The listing builds one solid part. Answer for the finished solid, in the listing's coordinates (mm). Face numbers are marked on the shaded views. A direction names the side the tool comes from. Coordinates: 2 decimals unless noted, no trailing zeros. Order: outer loops, then holes, each group sorted by start corner. A loop starts at its lowest first (then second) coordinate and runs counter-clockwise, first axis right, second up. Notation, with made-up numbers: (-13.75, 2.25) -> (13.25, 2.25) arc R22 cw to (13.25, 9.25) -> close; hole circle Ø4 at (76, 5). An arc over 180 degrees is marked (long way). One line per question, with ' | ' between items.
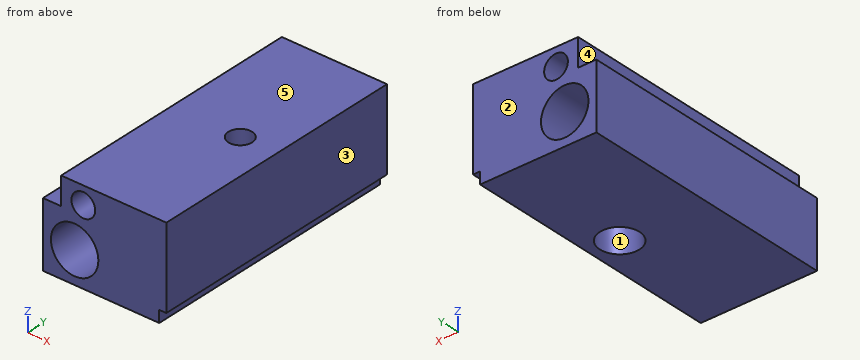
from build123d import *

# Parameters (mm, degrees)
F0_R          = 3
F0_R_2        = 1.5
F1_DEPTH      = 16.5
F1_DEPTH_BACK = 16.5
F2_R          = 1.5
F2_R_2        = 2.5
F3_DEPTH      = 6.5
F4_DEPTH      = 11.8


with BuildPart() as f1:
    # F0 (on Front) → F1 (new body, two sides)
    with BuildSketch(Plane.XZ) as f1_sk:
        Polygon((0, 8.3), (0, 0), (14.7, 0), (14.7, 1.5), (15.6, 1.5), (15.6, 11.8), (2.3, 11.8), (2.3, 8.3), align=None)
        with Locations((4, 4)):
            Circle(F0_R, mode=Mode.SUBTRACT)
        with Locations((5.1, 9.55)):
            Circle(F0_R_2, mode=Mode.SUBTRACT)
    extrude(amount=F1_DEPTH)
    extrude(f1_sk.sketch, amount=-F1_DEPTH_BACK)

    # F2 (on face) → F3 (cut)
    with BuildSketch(Plane(origin=(0, 0, 0), x_dir=(1, 0, 0), z_dir=(0, 0, -1))):
        with Locations((11, 0)):
            Circle(F2_R)
        with Locations((11, 0)):
            Circle(F2_R_2)
        with Locations((11, 0)):
            Circle(F2_R, mode=Mode.SUBTRACT)
    extrude(amount=-F3_DEPTH, mode=Mode.SUBTRACT)

    # F2 (on face) → F4 (cut, through all)
    with BuildSketch(Plane(origin=(0, 0, 0), x_dir=(1, 0, 0), z_dir=(0, 0, -1))):
        with Locations((11, 0)):
            Circle(F2_R)
    extrude(amount=-F4_DEPTH, mode=Mode.SUBTRACT)


solid = f1.part
Item 1: For the marked faces 4 and 5, determine the directions among +Z, -Z, +X, -X, +Y, -Y from which every point of the face is accessible in a straight line to the end or side of a thin tool.
Computed values:
face 4: +Z, -X, +Y, -Y | face 5: +Z, +X, -X, +Y, -Y
Item 2: Section C-C, the plane y = -1 is taken. Give the vertices of the cut face in (x, z), plus the area to 3 significant figures.
Computed values:
outline: (0, 0) -> (8.71, 0) -> (8.71, 6.5) -> (9.88, 6.5) -> (9.88, 11.8) -> (2.3, 11.8) -> (2.3, 8.3) -> (0, 8.3) -> close; (12.12, 6.5) -> (13.29, 6.5) -> (13.29, 0) -> (14.7, 0) -> (14.7, 1.5) -> (15.6, 1.5) -> (15.6, 11.8) -> (12.12, 11.8) -> close; hole circle Ø6 at (4, 4); hole circle Ø3 at (5.1, 9.55) | area: 97.7 mm^2
Item 3: Section B-B, the plane x = 11 is taken. Give the vertices of the cut face in (y, z), plus the area to 3 significant figures.
Computed values:
outline: (-16.5, 0) -> (-2.5, 0) -> (-2.5, 6.5) -> (-1.5, 6.5) -> (-1.5, 11.8) -> (-16.5, 11.8) -> close; (1.5, 6.5) -> (2.5, 6.5) -> (2.5, 0) -> (16.5, 0) -> (16.5, 11.8) -> (1.5, 11.8) -> close | area: 341 mm^2
Item 4: Section D-D, the plane x = 5 is taken. Give the vertices of the cut face in (y, z), plus the area to 3 significant figures.
Computed values:
outline: (-16.5, 0) -> (16.5, 0) -> (16.5, 1.17) -> (-16.5, 1.17) -> close; (-16.5, 6.83) -> (16.5, 6.83) -> (16.5, 8.05) -> (-16.5, 8.05) -> close; (-16.5, 11.05) -> (16.5, 11.05) -> (16.5, 11.8) -> (-16.5, 11.8) -> close | area: 104 mm^2
Item 5: Section A-A, the plane z = 4 is taken. Give the vertices of the cut face in (x, y), plus the area to 3 significant figures.
Computed values:
outline: (0, -16.5) -> (1, -16.5) -> (1, 16.5) -> (0, 16.5) -> close; (7, -16.5) -> (15.6, -16.5) -> (15.6, 16.5) -> (7, 16.5) -> close; hole circle Ø5 at (11, 0) | area: 297 mm^2
Item 6: Find the intervals of material crossed by L1, parallel to Z at x = 5.1, y = 9.75; L2, parallel to Z at x = 4, y = -7.5; L3, parallel to X at y = 0, z = 8.65, in increasing order.
Computed values:
L1: z = 0 to 1.21, 6.79 to 8.05, 11.05 to 11.8 | L2: z = 0 to 1, 7 to 8.53, 10.57 to 11.8 | L3: x = 2.3 to 3.9, 6.3 to 9.5, 12.5 to 15.6
Item 7: Each of these flat-tipped pins is pushed along its axis until it touches: pin 1 Ø0.7 at (x, y) = (1.5, -0.5) entering from +Z; pin 2 Ø1.8 at (y, z) = (-3.5, 9.5) entering from -X. Where does it stop, or does it pass through?
Computed values:
pin 1: stops at z = 8.3 | pin 2: stops at x = 2.3
Item 8: Determine the mould class of the marked faces 1, 2 and 3 for opening direction Y: pulls with the +Y half, pulls with the -Y half, needs draft (parallel to the pull), parting line crosses it, or undercut.
Computed values:
face 1: undercut | face 2: pulls with the +Y half | face 3: needs draft
